Can you work these out from the drawing? Everything is in mm from the part's minimum corner. A direction names the side the tool comes from. Give positions to 0.01 mm unless a question says otherwise; leave off trailing zeros. Loops run counter-clockwise (first coordinate to the right, second up) from the corner with the lowest first, then second, coordinate; pieces in that order, holes last.
Q1. We'd pull the mould along Y, two halves only. Please class the marked faces 4, 5, 6 and 7: +Y half, -Y half, draft (parallel to the pull), parting line (faces both ways), or undercut.
Q2. If we section it at D-D (x = 40.5): Please give me the cut outline in (y, z), plus the area to 3 significant figures.
Q3. For the marked faces 1, 2 and 3, which set-ups out of +Z, -Z, +X, -X, +Y, -Y let a thin tool reach every point of the face, with its end or its side?
Q4. I need wall thicknesses on line 1 (Y direction, x = 22, z = 6.5); line 2 (X direction, y = 12, z = 6.75); line 3 (Y direction, x = 41, z = 7.5). Which ranges of each line are inside material? Lowest first, please.
Q5. Will these pins go through, and if not, where does the flat tip stop? P1, Ø3, axis at x = 40, z = 7.5, coming from the +Y side; P2, Ø1.5, axis at x = 29.5, z = 5, coming from the -Y side; P3, Ø4, axis at y = 29, z = 9, coming from the +X side; P4, Ø3, axis at y = 14, z = 7, coming from the +X side.
Q6. If we section it at B-B (z = 6.75): Please give me the cut outline in (x, y).
Q7. If we section it at A-A (x = 22): Please give me the cut outline in (y, z).
Q8. If we section it at C-C (y = 15.5): Please give me the cut outline in (x, z).
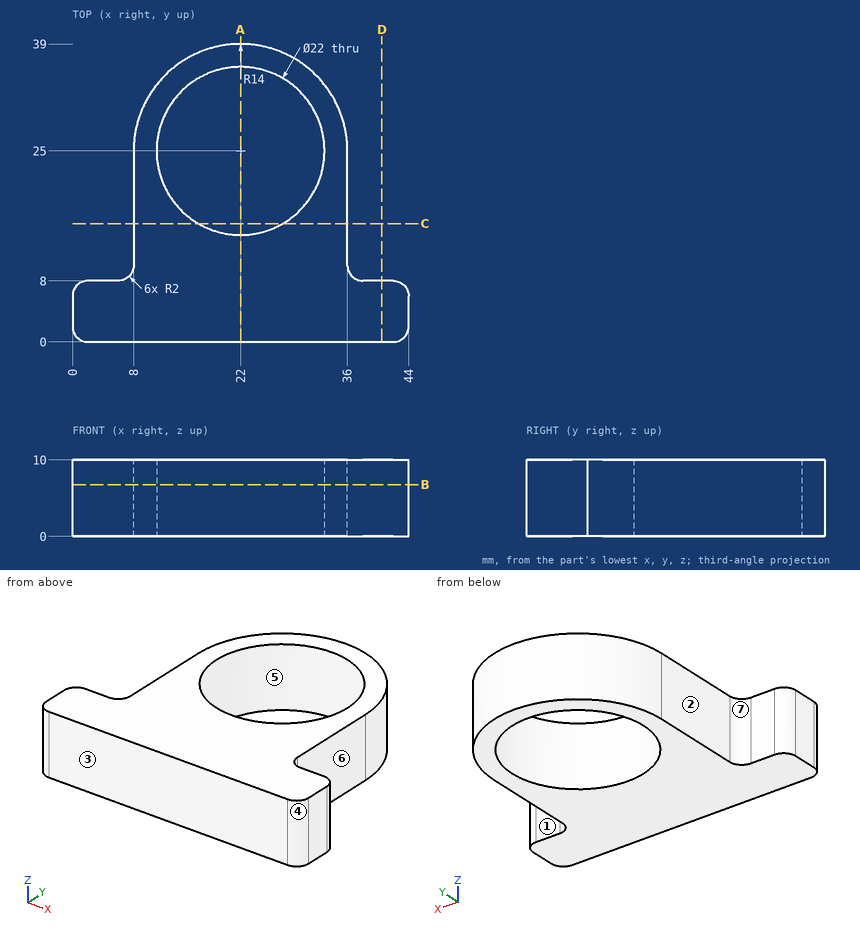
Check sheet entries:
1. face 4: -Y half
1. face 5: undercut
1. face 6: draft
1. face 7: +Y half
2. outline: (0, 0) - (8, 0) - (8, 10) - (0, 10) - close
2. area: 80.0 mm2
3. face 1: +Z, -Z, +X, +Y
3. face 2: +Z, -Z, -X, +Y
3. face 3: +Z, -Z, +X, -X, -Y
4. line 1: y = 0 to 14, 36 to 39
4. line 2: x = 8 to 36
4. line 3: y = 0 to 8
5. P1: stops at y = 8
5. P2: stops at y = 0
5. P3: stops at x = 35.86
5. P4: stops at x = 36
6. outline: (0, 2) arc R2 ccw to (2, 0) - (42, 0) arc R2 ccw to (44, 2) - (44, 6) arc R2 ccw to (42, 8) - (38, 8) arc R2 cw to (36, 10) - (36, 25) arc R14 ccw to (8, 25) - (8, 10) arc R2 cw to (6, 8) - (2, 8) arc R2 ccw to (0, 6) - close; hole circle Ø22 at (22, 25)
7. outline: (0, 0) - (14, 0) - (14, 10) - (0, 10) - close; (36, 0) - (39, 0) - (39, 10) - (36, 10) - close
8. outline: (8, 0) - (16.45, 0) - (16.45, 10) - (8, 10) - close; (27.55, 0) - (36, 0) - (36, 10) - (27.55, 10) - close
